Could you check a few things on this model? Use its own coordinates, in mm. Face numbers are marked on the shaded views. A direction names the side the tool comes from. Round coordinates to 2 decimals unless told otherwise and drop trailing zeros. Write each loop counter-clockwise with the first axis right and the second up, starting at its lowest first coordinate (ties: lowest second). Pieces come first, ordered by that corner, then holes. Notation, with made-up numbers: (-13.75, -5.75) -> (7.25, -5.75) arc R17 ccw to (7.25, 9.25) -> close; hole circle Ø1 at (40, 15.5). An arc over 180 degrees is marked (long way). Return JSON: item names as keys, results as strings.
from build123d import *

# Parameters (mm, degrees)
SKETCH_1_R          = 15.915
EXTRUDE_1_DEPTH     = 11
SKETCH_2_R          = 17
EXTRUDE_2_DEPTH     = 1
EXTRUDE_START       = 1
SKETCH_3_R          = 17
EXTRUDE_3_DEPTH     = 1
SKETCH_4_R          = 5
CUT_EXTRUDE_1_DEPTH = 28.331300737
EXTRUDE_START_2     = 10
SKETCH_5_R          = 12.5
SKETCH_5_R_2        = 5
EXTRUDE_4_DEPTH     = 10


with BuildPart() as part:
    # 草图1 → 凸台-拉伸1 (new body)
    with BuildSketch(Plane(origin=(0, 0, 0), x_dir=(1, 0, 0), z_dir=(0, 1, 0))):
        with Locations(Location((0, 0, 0), (0, 0, 270))):
            Circle(SKETCH_1_R)
    extrude(amount=EXTRUDE_1_DEPTH)

    # 草图2 → 凸台-拉伸2 (add)
    with BuildSketch(Plane(origin=(0, 11, 0), x_dir=(1, 0, 0), z_dir=(0, 1, 0))):
        with Locations(Location((0, 0, 0), (0, 0, 270))):
            Circle(SKETCH_2_R)
    extrude(amount=EXTRUDE_2_DEPTH)

    # 草图3 → 凸台-拉伸3 (add)
    with BuildSketch(Plane.XZ.offset(EXTRUDE_START)):
        with Locations(Location((0, 0, 0), (0, 0, 90))):
            Circle(SKETCH_3_R)
    extrude(amount=-EXTRUDE_3_DEPTH)

    # 草图4 → 切除-拉伸1 (cut, through all)
    with BuildSketch(Plane.XZ.offset(1)):
        with Locations(Location((0, 0, 0), (0, 0, 270))):
            Circle(SKETCH_4_R)
    extrude(amount=-CUT_EXTRUDE_1_DEPTH, mode=Mode.SUBTRACT)

    # 草图5 → 凸台-拉伸4 (add)
    with BuildSketch(Plane.XZ.offset(1).offset(EXTRUDE_START_2)):
        with Locations(Location((0, 0, 0), (0, 0, 270))):
            Circle(SKETCH_5_R)
        with Locations(Location((0, 0, 0), (0, 0, 270))):
            Circle(SKETCH_5_R_2, mode=Mode.SUBTRACT)
    extrude(amount=-EXTRUDE_4_DEPTH)


solid = part.part
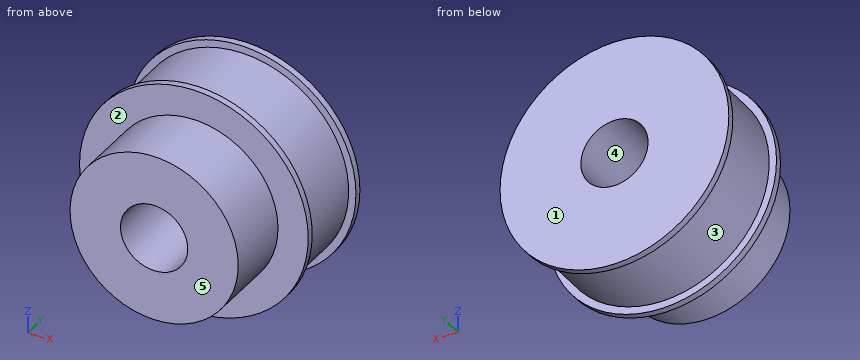
1) For the marked faces 1 and 2, which set-ups out of +Z, -Z, +X, -X, +Y, -Y let a thin tool reach every point of the face, with its end or its side?
Return value:
{"face 1": "+Z, -Z, +X, -X, +Y", "face 2": "-Y"}
2) I want a section at D-D, the plane z = -13.5. Please give me the cut outline in (x, y), and give its area (3 significant figures).
Return value:
{"outline": "(-10.33, -1) -> (10.33, -1) -> (10.33, 0) -> (8.43, 0) -> (8.43, 11) -> (10.33, 11) -> (10.33, 12) -> (-10.33, 12) -> (-10.33, 11) -> (-8.43, 11) -> (-8.43, 0) -> (-10.33, 0) -> close", "area": "227 mm²"}
3) Thinking about a two-plate mould opening in Z: for the marked faces 3, 4 and 5, which applies, pulls with the +Z half, pulls with the -Z half, needs draft (parallel to the pull), parting line crosses it, or undercut?
Return value:
{"face 3": "parting line crosses it", "face 4": "undercut", "face 5": "needs draft"}
4) I want a section at A-A, the plane x = 0. Please give me the cut outline in (y, z) (3 decimals).
Return value:
{"outline": "(-11, -12.5) -> (-1, -12.5) -> (-1, -17) -> (0, -17) -> (0, -15.915) -> (11, -15.915) -> (11, -17) -> (12, -17) -> (12, -5) -> (-11, -5) -> close; (-11, 5) -> (12, 5) -> (12, 17) -> (11, 17) -> (11, 15.915) -> (0, 15.915) -> (0, 17) -> (-1, 17) -> (-1, 12.5) -> (-11, 12.5) -> close"}
5) I want a section at C-C, the plane y = 1. Please give me the cut outline in (x, z) (3 decimals), and give its area (3 significant figures).
Return value:
{"outline": "circle Ø31.83 at (0, 0); hole circle Ø10 at (0, 0)", "area": "717 mm²"}
6) If I drill on probe 1 along X at (y, z) = (1, 0) (3 decimals); probe 2 along X at (y, z) = (-3.75, 0); probe 3 along Y at (x, z) = (-8.5, -12), over which ranges is the centre line in solid material (lowest first)? Write a range as [from, to].
Return value:
{"probe 1": "[-15.915, -5], [5, 15.915]", "probe 2": "[-12.5, -5], [5, 12.5]", "probe 3": "[-1, 12]"}
7) Will these pins go through, and if not, where does the flat tip stop? pin 1 Ø4 at (x, y) = (-6, -7.5) entering from -Z; pin 2 Ø5 at (x, y) = (4, -1.5) entering from +Z; pin 3 Ø10 at (y, z) = (2.5, -5.5) entering from +X.
Return value:
{"pin 1": "z = -11.84", "pin 2": "z = 16.93", "pin 3": "x = 16.96"}
8) I want a section at B-B, the plane z = 0. Please give me the cut outline in (x, y) (3 decimals).
Return value:
{"outline": "(-17, -1) -> (-12.5, -1) -> (-12.5, -11) -> (-5, -11) -> (-5, 12) -> (-17, 12) -> (-17, 11) -> (-15.915, 11) -> (-15.915, 0) -> (-17, 0) -> close; (5, -11) -> (12.5, -11) -> (12.5, -1) -> (17, -1) -> (17, 0) -> (15.915, 0) -> (15.915, 11) -> (17, 11) -> (17, 12) -> (5, 12) -> close"}
